```python
from build123d import *

# Parameters (mm, degrees)
SKETCH_1_R          = 5
SKETCH_1_R_2        = 1.5
EXTRUDE_1_DEPTH     = 25
SKETCH_2_R          = 2.15
CUT_EXTRUDE_1_DEPTH = 30
SKETCH_3_R          = 2.15
CUT_EXTRUDE_2_DEPTH = 30
SKETCH_4_W          = 34
SKETCH_4_H          = 42.25
CUT_EXTRUDE_3_DEPTH = 15
CHAMFER_1_SIZE      = 5
CHAMFER_2_SIZE      = 3
SKETCH_6_R          = 9.75
CUT_EXTRUDE_5_DEPTH = 6.2
EXTRUDE_2_DEPTH     = 5
SKETCH_8_W          = 91.561993536
SKETCH_8_H          = 85.949306993
CUT_EXTRUDE_6_DEPTH = 25
CHAMFER_3_SIZE      = 8
SKETCH_9_R          = 1.5
CUT_EXTRUDE_7_DEPTH = 10
SKETCH_10_R         = 1.5
CUT_EXTRUDE_8_DEPTH = 5


with BuildPart() as part:
    # 草图1 → 凸台-拉伸1 (new body)
    with BuildSketch(Plane.XY):
        Polygon((0, 0), (0, 20), (20, 20), (20, 25), (0, 25), (0, 67.25), (-34, 67.25), (-34, 20), (-5, 20), (-5, 0), align=None)
        with Locations((-17, 50.25)):
            Circle(SKETCH_1_R, mode=Mode.SUBTRACT)
        with Locations((-29, 62.25)):
            Circle(SKETCH_1_R_2, mode=Mode.SUBTRACT)
        with Locations((-5, 62.25)):
            Circle(SKETCH_1_R_2, mode=Mode.SUBTRACT)
        with Locations((-29, 38.25)):
            Circle(SKETCH_1_R_2, mode=Mode.SUBTRACT)
        with Locations((-5, 38.25)):
            Circle(SKETCH_1_R_2, mode=Mode.SUBTRACT)
    extrude(amount=EXTRUDE_1_DEPTH)

    # 草图2 → 切除-拉伸1 (cut)
    with BuildSketch(Plane(origin=(0, 0, 0), x_dir=(0, 0, -1), z_dir=(1, 0, 0))):
        with Locations((-12.5, 10)):
            Circle(SKETCH_2_R)
    extrude(amount=-CUT_EXTRUDE_1_DEPTH, mode=Mode.SUBTRACT)

    # 草图3 → 切除-拉伸2 (cut)
    with BuildSketch(Plane.XZ.offset(-20)):
        with Locations(Location((10, 12.5, 0), (0, 0, 270))):
            Circle(SKETCH_3_R)
    extrude(amount=-CUT_EXTRUDE_2_DEPTH, mode=Mode.SUBTRACT)

    # 草图4 → 切除-拉伸3 (cut)
    with BuildSketch(Plane(origin=(0, 0, 0), x_dir=(-1, 0, 0), z_dir=(0, 0, -1))):
        with Locations((17, 46.125)):
            Rectangle(SKETCH_4_W, SKETCH_4_H)
    extrude(amount=-CUT_EXTRUDE_3_DEPTH, mode=Mode.SUBTRACT)

    # 倒角1
    chamfer_1_edges = [part.edges().sort_by_distance(p)[0] for p in [
        (-5, 20, 12.5),
        (0, 25, 20),
    ]]
    chamfer(chamfer_1_edges, length=CHAMFER_1_SIZE)

    # 倒角2
    chamfer_2_edges = [part.edges().sort_by_distance(p)[0] for p in [
        (-34, 67.25, 20),
        (0, 67.25, 20),
    ]]
    chamfer(chamfer_2_edges, length=CHAMFER_2_SIZE)

    # 草图6 → 切除-拉伸5 (cut)
    with BuildSketch(Plane(origin=(0, 0, 15), x_dir=(-1, 0, 0), z_dir=(0, 0, -1))):
        with Locations((17, 50.25)):
            Circle(SKETCH_6_R)
    extrude(amount=-CUT_EXTRUDE_5_DEPTH, mode=Mode.SUBTRACT)

    # 草图7 → 凸台-拉伸2 (add)
    with BuildSketch(Plane.XY.offset(25)):
        Polygon((-34, 20), (-10, 20), (-5, 15), (-5, 0), align=None)
    extrude(amount=-EXTRUDE_2_DEPTH)


with BuildPart() as body_2:
    # 镜向1: mirrored copy
    add(part.part.mirror(Plane.XY.offset(25)))

    # 倒角3
    # the kernel refuses this chamfer: 8 mm, written as the material it adds along each edge
    with BuildSketch(Plane(origin=(-34, 25, 35), x_dir=(0, 0.9996219169112968, -0.027495876610586487), z_dir=(1, 0, 0))) as chamfer_3_piece_1_section:
        Polygon((CHAMFER_3_SIZE * 0.999621916911, CHAMFER_3_SIZE * 0.0274958766106), (-CHAMFER_3_SIZE * 0.0274958766106, CHAMFER_3_SIZE * 0.999621916911), (0, 0), align=None)
    chamfer_3_piece_1 = extrude(amount=59.573463904, mode=Mode.PRIVATE)
    chamfer_3_piece_1 = split(chamfer_3_piece_1, bisect_by=Plane(origin=(0, 27.617876763, 37.64907513), z_dir=(-1, 0, 0)), keep=Keep.TOP, mode=Mode.PRIVATE)
    chamfer_3_piece_1 = split(chamfer_3_piece_1, bisect_by=Plane(origin=(-7.349818702, 37.349818702, 37.64907513), z_dir=(-0.7071067811865476, -0.7071067811865476, 0)), keep=Keep.TOP, mode=Mode.PRIVATE)
    add(chamfer_3_piece_1)
    with BuildSketch(Plane(origin=(-34, 25, 35), x_dir=(0, 0.9996219169112968, -0.027495876610586487), z_dir=(1, 0, 0))) as chamfer_3_piece_2_section:
        Polygon((CHAMFER_3_SIZE * 0.999621916911, CHAMFER_3_SIZE * 0.0274958766106), (-CHAMFER_3_SIZE * 0.0274958766106, CHAMFER_3_SIZE * 0.999621916911), (0, 0), align=None)
    chamfer_3_piece_2 = extrude(amount=59.573463904, mode=Mode.PRIVATE)
    chamfer_3_piece_2 = split(chamfer_3_piece_2, bisect_by=Plane(origin=(0, 26.307184644, 38.352912701), z_dir=(1, 0, 0)), keep=Keep.TOP, mode=Mode.PRIVATE)
    chamfer_3_piece_2 = split(chamfer_3_piece_2, bisect_by=Plane(origin=(2.769611517, 27.230388483, 38.352912701), z_dir=(-0.7071067811865476, -0.7071067811865476, 0)), keep=Keep.TOP, mode=Mode.PRIVATE)
    add(chamfer_3_piece_2)
    with BuildSketch(Plane(origin=(-34, 25, 35), x_dir=(0, 0.9996219169112968, -0.027495876610586487), z_dir=(1, 0, 0))) as chamfer_3_piece_3_section:
        Polygon((CHAMFER_3_SIZE * 0.999621916911, CHAMFER_3_SIZE * 0.0274958766106), (-CHAMFER_3_SIZE * 0.0274958766106, CHAMFER_3_SIZE * 0.999621916911), (0, 0), align=None)
    chamfer_3_piece_3 = extrude(amount=59.573463904, mode=Mode.PRIVATE)
    chamfer_3_piece_3 = split(chamfer_3_piece_3, bisect_by=Plane(origin=(0, 31.684169789, 35.518604569), z_dir=(-1, 0, 0)), keep=Keep.TOP, mode=Mode.PRIVATE)
    chamfer_3_piece_3 = split(chamfer_3_piece_3, bisect_by=Plane(origin=(-1.263127342, 31.263127342, 35.518604569), z_dir=(0.7071067811865476, 0.7071067811865476, 0)), keep=Keep.TOP, mode=Mode.PRIVATE)
    add(chamfer_3_piece_3)

    # 草图9 → 切除-拉伸7 (cut)
    with BuildSketch(Plane.ZY.offset(34)):
        with Locations(Location((40, 24, 0), (0, 0, 270))):
            Circle(SKETCH_9_R)
        with Locations(Location((32, 24, 0), (0, 0, 270))):
            Circle(SKETCH_9_R)
    extrude(amount=-CUT_EXTRUDE_7_DEPTH, mode=Mode.SUBTRACT)

    # 草图10 → 切除-拉伸8 (cut)
    with BuildSketch(Plane(origin=(0, 67.25, 0), x_dir=(1, 0, 0), z_dir=(0, 1, 0))):
        with Locations(Location((-12, -30, 0), (0, 0, 270))):
            Circle(SKETCH_10_R)
        with Locations(Location((-20, -30, 0), (0, 0, 270))):
            Circle(SKETCH_10_R)
    extrude(amount=-CUT_EXTRUDE_8_DEPTH, mode=Mode.SUBTRACT)


with BuildPart() as part_1:
    add(part.part)

    # 草图8 → 切除-拉伸6 (cut)
    with BuildSketch(Plane(origin=(0, 0, 0), x_dir=(-1, 0, 0), z_dir=(0, 0, -1))):
        with Locations((16.502686865, 35.124779943)):
            Rectangle(SKETCH_8_W, SKETCH_8_H)
    extrude(amount=-CUT_EXTRUDE_6_DEPTH, mode=Mode.SUBTRACT)


solid = body_2.part
```
Read the model definition and answer for the solid it produces. Units are mm, in the model's axes. A direction names the side the tool comes from. Round coordinates to 2 decimals unless told otherwise and drop trailing zeros. Write each loop counter-clockwise with the first axis right and the second up, starting at its lowest first coordinate (ties: lowest second). Pieces come first, ordered by that corner, then holes. Notation, with made-up numbers: (-21.75, 32.5) - (3.25, 32.5) arc R20 ccw to (3.25, 71.5) - close; hole circle Ø10 at (23, -31.75). An arc over 180 degrees is marked (long way). Use CSV: the item, a comma, the result in double quotes.
Q1. Each of these flat-tipped pins is pushed along its axis until it touches: pin 1 Ø1.5 at (y, z) = (24, 32) entering from -X; pin 2 Ø2.5 at (x, z) = (-20, 30) entering from +Y; pin 3 Ø4 at (y, z) = (51, 31.5) entering from +X. Where does it stop, or does it pass through?
Values:
pin 1,"stops at x = -24"
pin 2,"stops at y = 62.25"
pin 3,"stops at x = 0"
Q2. A tool of negligible diameter and unlimited length cuts with its end or side. For faces 4 (the cylindrical face through (-29.07, 24.325, 30.536)), 5 (the flat face through (-15, 55, 28.8)), 6 (the flat face through (-24, 43, 35)), 7 (the flat face through (-20, 62.25, 30)), from which of +Z, -Z, +X, -X, +Y, -Y can it reach the whole face along a straight path? Write none if from no direction.
Values:
face 4,"-X"
face 5,"+Z"
face 6,"+Z, +X, -X, +Y"
face 7,"+Y"
Q3. Straight lines are drawn through the part: line 1 along X through (y, z) = (38.25, 31); line 2 along Z through (x, y) = (-31, 24); line 3 along Y through (x, z) = (-16.5, 32.5). For each, find the intervals that lie inside material, in ascending order.
Values:
line 1,"x = -34 to -30.5, -27.5 to -6.5, -3.5 to 0"
line 2,"z = 25 to 30.5, 33.5 to 38.5, 41.5 to 50"
line 3,"y = 20 to 40.51, 59.99 to 67.25"
Q4. Find section C-C, the plane x = -29. Write down the section's boundary in (y, z).
Values:
outline,"(16.55, 25) - (36.75, 25) - (36.75, 35) - (33, 35) - (25, 43) - (25, 50) - (20, 50) - (20, 30) - (16.55, 30) - close; (39.75, 25) - (60.75, 25) - (60.75, 35) - (39.75, 35) - close; (63.75, 25) - (67.25, 25) - (67.25, 35) - (63.75, 35) - close; hole circle Ø3 at (24, 32); hole circle Ø3 at (24, 40)"
Q5. Find section B-B, the plane x = 10. Write down the section's boundary in (y, z).
Values:
outline,"(20, 25) - (25, 25) - (25, 35.35) - (20, 35.35) - close; (20, 39.65) - (25, 39.65) - (25, 50) - (20, 50) - close"
Q6. Find section D-D, the plane z = 47.5. Write down the section's boundary in (x, y), then the cut area to 4 significant figures.
Values:
outline,"(-34, 20) - (-10, 20) - (-5, 15) - (-5, 0) - (0, 0) - (0, 20) - (20, 20) - (20, 25) - (-34, 25) - close"
area,"382.5 mm²"
Q7. Determine the mould class of faces 1 (the cylindrical face through (-2.46, 10.65, 39.55)), 2 (the flat face through (-8, 18, 40)), 3 (the cylindrical face through (-14.89, 40.73, 31.94)) for opening direction X: +X half, -X half, draft (parallel to the pull), parting line (faces both ways), or undercut.
Values:
face 1,"draft"
face 2,"-X half"
face 3,"undercut"
Q8. Find section A-A, the plane y = 24. Write down the section's boundary in (x, z), then the cut area to 3 significant figures.
Values:
outline,"(-34, 25) - (20, 25) - (20, 50) - (-34, 50) - (-34, 41.5) - (-24, 41.5) - (-24, 38.5) - (-34, 38.5) - (-34, 33.5) - (-24, 33.5) - (-24, 30.5) - (-34, 30.5) - close; hole circle Ø4.3 at (10, 37.5)"
area,"1,280 mm²"
